```python
from build123d import *

# Parameters (mm, degrees)
EXTRUDE_1_DEPTH     = 3
CUT_EXTRUDE_1_DEPTH = 3
CUT_EXTRUDE_2_DEPTH = 3
SKETCH_5_R          = 1.5
CUT_EXTRUDE_3_DEPTH = 3
CUT_EXTRUDE_4_DEPTH = 3
SKETCH_7_R          = 7
CUT_EXTRUDE_5_DEPTH = 3
SKETCH_8_R          = 7
CUT_EXTRUDE_6_DEPTH = 10


with BuildPart() as part:
    # 草图1 → 凸台-拉伸1 (new body)
    with BuildSketch(Plane.XY):
        with BuildLine():
            Line((34, 0), (42.481679801, -249.85608079))
            Line((42.481679801, -249.85608079), (-25.518320199, -249.85608079))
            Line((-25.518320199, -249.85608079), (-34, 0))
            ThreePointArc((-34, 0), (0, 34), (34, 0))
        make_face()
    extrude(amount=EXTRUDE_1_DEPTH)

    # 草图3 → 切除-拉伸1 (cut)
    with BuildSketch(Plane.XY.offset(3)):
        with BuildLine():
            Line((-12.172192567, -230.017175725), (-34, 0))
            Line((-34, 0), (-25.518320199, -249.85608079))
            Line((-25.518320199, -249.85608079), (5.294460669, -249.85608079))
            ThreePointArc((5.294460669, -249.85608079), (-7.18330404, -243.233322379), (-12.172192567, -230.017175725))
        make_face()
    extrude(amount=-CUT_EXTRUDE_1_DEPTH, mode=Mode.SUBTRACT)

    # 草图3<4> → 切除-拉伸2 (cut)
    with BuildSketch(Plane.XY.offset(3)):
        with BuildLine():
            Line((42.481679801, -249.85608079), (34, 0))
            Line((34, 0), (27.827807433, -230.017175725))
            ThreePointArc((27.827807433, -230.017175725), (22.838918905, -243.233322379), (10.361154196, -249.85608079))
            Line((10.361154196, -249.85608079), (42.481679801, -249.85608079))
        make_face()
    extrude(amount=-CUT_EXTRUDE_2_DEPTH, mode=Mode.SUBTRACT)

    # 草图5 → 切除-拉伸3 (cut)
    with BuildSketch(Plane.XY.offset(3)):
        with Locations((0, 22)):
            Circle(SKETCH_5_R)
        with Locations((0, 15)):
            Circle(SKETCH_5_R)
        with Locations((-22, 0)):
            Circle(SKETCH_5_R)
        with Locations((-15, 0)):
            Circle(SKETCH_5_R)
        with Locations((0, -15)):
            Circle(SKETCH_5_R)
        with Locations((15, 0)):
            Circle(SKETCH_5_R)
        with Locations((22, 0)):
            Circle(SKETCH_5_R)
        with Locations((0, -22)):
            Circle(SKETCH_5_R)
    extrude(amount=-CUT_EXTRUDE_3_DEPTH, mode=Mode.SUBTRACT)

    # 草图6 → 切除-拉伸4 (cut)
    with BuildSketch(Plane.XY.offset(3)):
        Polygon((0, -34), (-10.183472327, -133.231632376), (4.42204079, -155.940198746), (18.166966985, -132.700641867), align=None)
    extrude(amount=-CUT_EXTRUDE_4_DEPTH, mode=Mode.SUBTRACT)

    # 草图7 → 切除-拉伸5 (cut)
    with BuildSketch(Plane.XY.offset(3)):
        with Locations((7.827807433, -230.017175725)):
            Circle(SKETCH_7_R)
    extrude(amount=-CUT_EXTRUDE_5_DEPTH, mode=Mode.SUBTRACT)

    # 草图8 → 切除-拉伸6 (cut)
    with BuildSketch(Plane.XY.offset(3)):
        Circle(SKETCH_8_R)
    extrude(amount=-CUT_EXTRUDE_6_DEPTH, mode=Mode.SUBTRACT)


solid = part.part
```
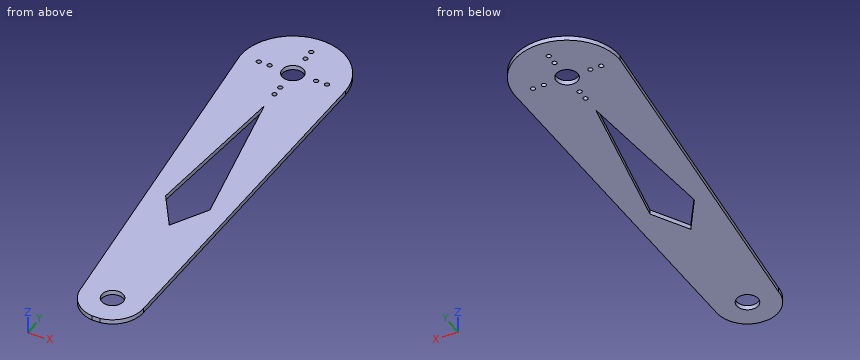
CAD build for the part. Positions are in the model's coordinates, mm. Coordinates: 2 decimals unless noted, no trailing zeros. Write each loop counter-clockwise with the first axis right and the second up, starting at its lowest first coordinate (ties: lowest second). Pieces come first, ordered by that corner, then holes.
(1) Drill centre lines: probe 1 along X at (y, z) = (3, 1.9); probe 2 along Y at (x, z) = (22, 2.3); probe 3 along X at (y, z) = (22.5, 1.45). Where is each one in solid material? Low to high.
(2) Cut at B-B, the plane y = -150. List the corners of the cut face in (x, z), and give its area (3 significant figures).
(3) Cut at D-D, the plane y = -186. List the corners of the cut face in (x, z).
(4) Flat gauge pins, fed straight in: pin 1 (1.5 mm diameter, centred on x = 27, z = 1.5, fed in from +Y); pin 2 (1.5 mm diameter, centred on x = -21, z = 1, fed in from +Y); pin 3 (1 mm diameter, centred on x = 9.5, z = 1.5, fed in from +Y). Where does each tip first touch, or does it go through?
(5) Cut at C-C, the plane y = -80. List the corners of the cut face in (x, z).
(6) Cut at A-A, the plane z = 1. Count the separate pieces of the cut face and the enclosed holes in it, and give its area (3 significant figures).
Geometry says:
1. probe 1: x = -33.87 to -6.32, 6.32 to 33.87
1. probe 2: y = -244.13 to -1.5, 1.5 to 25.92
1. probe 3: x = -25.49 to -1.41, 1.41 to 25.49
2. outline: (-19.77, 0) - (0.6, 0) - (0.6, 3) - (-19.77, 3) - close; (7.94, 0) - (29.97, 0) - (29.97, 3) - (7.94, 3) - close
2. area: 127 mm2
3. outline: (-16.35, 0) - (29.01, 0) - (29.01, 3) - (-16.35, 3) - close
4. pin 1: stops at y = 21.61
4. pin 2: stops at y = 27.31
4. pin 3: stops at y = 32.79
5. outline: (-26.41, 0) - (-4.72, 0) - (-4.72, 3) - (-26.41, 3) - close; (8.47, 0) - (31.85, 0) - (31.85, 3) - (8.47, 3) - close
6. separate pieces: 1
6. enclosed holes: 11
6. area: 12,800 mm2
